Geometry: final body of the model. Coordinates: model frame, mm. A direction names the side the tool comes from. Give positions to 0.01 mm unless a question says otherwise; leave off trailing zeros. Loops run counter-clockwise (first coordinate to the right, second up) from the corner with the lowest first, then second, coordinate; pieces in that order, holes last.
from build123d import *

# Parameters (mm, degrees)
BOSS_EXTRUDE1_DEPTH = 20.5
SKETCH2_W           = 6
SKETCH2_H           = 13
SKETCH2_W_2         = 25
SKETCH2_H_2         = 6
CUT_EXTRUDE1_DEPTH  = 8
SKETCH3_W           = 23
SKETCH3_H           = 23
BOSS_EXTRUDE2_DEPTH = 7
SKETCH4_W           = 31
SKETCH4_H           = 32.5
SKETCH4_W_2         = 23
SKETCH4_H_2         = 23
BOSS_EXTRUDE4_DEPTH = 19
CUT_EXTRUDE2_REACH  = 53.403
SKETCH5_W           = 2.6
SKETCH5_H           = 5.5
SKETCH5_H_2         = 4
SKETCH5_W_2         = 4
SKETCH5_H_3         = 15
SKETCH5_W_3         = 2
SKETCH6_R           = 1.5
CUT_EXTRUDE3_DEPTH  = 10
SKETCH7_W           = 8
SKETCH7_H           = 9
BOSS_EXTRUDE5_DEPTH = 20.5
SKETCH8_R           = 2
CUT_EXTRUDE4_DEPTH  = 10


with BuildPart() as part:
    # Sketch1 → Boss-Extrude1 (new body)
    with BuildSketch(Plane(origin=(0, 0, 0), x_dir=(1, 0, 0), z_dir=(0, 1, 0))):
        Polygon((29, -32.5), (35, -32.5), (35, 32.5), (-35, 32.5), (-35, -32.5), (-29, -32.5), (-29, 26.5), (29, 26.5), align=None)
    extrude(amount=BOSS_EXTRUDE1_DEPTH)

    # Sketch2 → Cut-Extrude1 (cut)
    with BuildSketch(Plane.XZ):
        with Locations((32, 26)):
            Rectangle(SKETCH2_W, SKETCH2_H)
        with Locations((0, -29.5)):
            Rectangle(SKETCH2_W_2, SKETCH2_H_2)
        with Locations((-32, 26)):
            Rectangle(SKETCH2_W, SKETCH2_H)
    extrude(amount=-CUT_EXTRUDE1_DEPTH, mode=Mode.SUBTRACT)



with BuildPart() as body_2:
    # Sketch3 → Boss-Extrude2 (new body)
    with BuildSketch(Plane(origin=(0, 20.5, 0), x_dir=(1, 0, 0), z_dir=(0, 1, 0))):
        with Locations((-2.5, 9.5)):
            Rectangle(SKETCH3_W, SKETCH3_H)
    extrude(amount=-BOSS_EXTRUDE2_DEPTH)


with BuildPart() as part_1:
    add(part.part)

    add(body_2.part)  # Boss-Extrude4 merges body 2
    # Sketch4 → Boss-Extrude4 (add)
    with BuildSketch(Plane(origin=(0, 20.5, 0), x_dir=(1, 0, 0), z_dir=(0, 1, 0))):
        with Locations((-2.5, 10.25)):
            Rectangle(SKETCH4_W, SKETCH4_H)
        with Locations((-2.5, 9.5)):
            Rectangle(SKETCH4_W_2, SKETCH4_H_2, mode=Mode.SUBTRACT)
    extrude(amount=-BOSS_EXTRUDE4_DEPTH)

    # Cut-Extrude2: up to this face of the body (flat: up to its plane)
    cut_extrude2_end = Plane(part_1.part.faces().sort_by_distance((-2.5, 13.5, -9.5))[0])
    # Sketch5 → Cut-Extrude2 (cut, up to the picked face)
    with BuildSketch(Plane.XZ.offset(-1.5), mode=Mode.PRIVATE) as cut_extrude2_sk1:
        with Locations((-8.25, -23.75)):
            Rectangle(SKETCH5_W, SKETCH5_H)
    cut_extrude2_tool1 = split(extrude(cut_extrude2_sk1.sketch, amount=-CUT_EXTRUDE2_REACH, mode=Mode.PRIVATE), bisect_by=cut_extrude2_end, keep=Keep.BOTH, mode=Mode.PRIVATE)
    # Sketch5 → Cut-Extrude2 (cut, up to the picked face)
    with BuildSketch(Plane.XZ.offset(-1.5), mode=Mode.PRIVATE) as cut_extrude2_sk2:
        with Locations((-8.25, 4)):
            Rectangle(SKETCH5_W, SKETCH5_H_2)
    cut_extrude2_tool2 = split(extrude(cut_extrude2_sk2.sketch, amount=-CUT_EXTRUDE2_REACH, mode=Mode.PRIVATE), bisect_by=cut_extrude2_end, keep=Keep.BOTH, mode=Mode.PRIVATE)
    # Sketch5 → Cut-Extrude2 (cut, up to the picked face)
    with BuildSketch(Plane.XZ.offset(-1.5), mode=Mode.PRIVATE) as cut_extrude2_sk3:
        with Locations((-16, -5.5)):
            Rectangle(SKETCH5_W_2, SKETCH5_H_3)
    cut_extrude2_tool3 = split(extrude(cut_extrude2_sk3.sketch, amount=-CUT_EXTRUDE2_REACH, mode=Mode.PRIVATE), bisect_by=cut_extrude2_end, keep=Keep.BOTH, mode=Mode.PRIVATE)
    # Sketch5 → Cut-Extrude2 (cut, up to the picked face)
    with BuildSketch(Plane.XZ.offset(-1.5), mode=Mode.PRIVATE) as cut_extrude2_sk4:
        with Locations((3.55, 4)):
            Rectangle(SKETCH5_W_3, SKETCH5_H_2)
    cut_extrude2_tool4 = split(extrude(cut_extrude2_sk4.sketch, amount=-CUT_EXTRUDE2_REACH, mode=Mode.PRIVATE), bisect_by=cut_extrude2_end, keep=Keep.BOTH, mode=Mode.PRIVATE)
    add(cut_extrude2_tool1.solids().sort_by(Axis((-8.25, 1.5, -23.75), (0, 1, 0)))[0], mode=Mode.SUBTRACT)
    add(cut_extrude2_tool2.solids().sort_by(Axis((-8.25, 1.5, 4), (0, 1, 0)))[0], mode=Mode.SUBTRACT)
    add(cut_extrude2_tool3.solids().sort_by(Axis((-16, 1.5, -5.5), (0, 1, 0)))[0], mode=Mode.SUBTRACT)
    add(cut_extrude2_tool4.solids().sort_by(Axis((3.55, 1.5, 4), (0, 1, 0)))[0], mode=Mode.SUBTRACT)

    # Sketch6 → Cut-Extrude3 (cut)
    with BuildSketch(Plane.XZ):
        with Locations(Location((-32, 14.5, 0), (0, 0, 270))):
            Circle(SKETCH6_R)
        with Locations(Location((-32, -21.5, 0), (0, 0, 270))):
            Circle(SKETCH6_R)
    cut_extrude3 = extrude(amount=-CUT_EXTRUDE3_DEPTH, mode=Mode.SUBTRACT)

    # Mirror1: Cut-Extrude3 across plane
    add(cut_extrude3.mirror(Plane(origin=(0, 0, 0), x_dir=(0, 0, 1), z_dir=(1, 0, 0))), mode=Mode.SUBTRACT)

    # Sketch7 → Boss-Extrude5 (add)
    with BuildSketch(Plane(origin=(0, 20.5, 0), x_dir=(1, 0, 0), z_dir=(0, 1, 0))):
        with Locations((25, 22)):
            Rectangle(SKETCH7_W, SKETCH7_H)
        with Locations((-25, 22)):
            Rectangle(SKETCH7_W, SKETCH7_H)
    extrude(amount=-BOSS_EXTRUDE5_DEPTH)

    # Sketch8 → Cut-Extrude4 (cut)
    with BuildSketch(Plane(origin=(0, 0, -32.5), x_dir=(-1, 0, 0), z_dir=(0, 0, -1))):
        with Locations((-25, 11)):
            Circle(SKETCH8_R)
        with Locations((25, 11)):
            Circle(SKETCH8_R)
    extrude(amount=-CUT_EXTRUDE4_DEPTH, mode=Mode.SUBTRACT)


solid = part_1.part
Item 1: Section query A-A on z = 17.5. Return loops of the section in (x, y), plus the area to 3 significant figures.
Values follow:
outline: (-35, 0) - (-29, 0) - (-29, 20.5) - (-35, 20.5) - close; (29, 0) - (35, 0) - (35, 20.5) - (29, 20.5) - close
area: 246 mm2
Item 2: Section query D-D on x = 3.5. Return loops of the section in (y, z), plus the area to 4 significant figures.
Values follow:
outline: (1.5, -26.5) - (8, -26.5) - (8, -32.5) - (20.5, -32.5) - (20.5, 6) - (13.5, 6) - (13.5, -21) - (1.5, -21) - close
area: 368.5 mm2
Item 3: Pin query (flat end, axial travel): pin 1 (2 mm diameter, centred on x = -8, y = 11, fed in from +Z); pin 2 (6 mm diameter, centred on x = -22.5, y = 11, fed in from +Z); pin 3 (8 mm diameter, centred on x = -6.5, z = -5.5, fed in from -Y); pin 4 (10.5 mm diameter, centred on x = -3.5, y = 5, fed in from -Z). Return the tip coordinate at first contact, or that it passes through.
Values follow:
pin 1: stops at z = -26.5
pin 2: stops at z = -17.5
pin 3: stops at y = 13.5
pin 4: stops at z = -32.5
Item 4: Set-up query: faces 4 (the face through (-25, 11, -22.5)), 5 (the face through (-14, 7, 2)), 6 (the face through (3, 5, -26.5)), 7 (the face through (-29, 10, 8)). Return all of +Z, -Z, +X, -X, +Y, -Y with unobstructed straight access to the full face (end or side cutting, diameter ignored); none if empty.
Values follow:
face 4: -Z
face 5: -Y
face 6: -Z, -Y
face 7: +Z, +Y, -Y
Item 5: Draft query along Z for faces 1 (the face through (12.5, 4, -30)), 2 (the face through (-32, 10, -21)), 3 (the face through (-32, 14, 32.5)). Return one class per face: +Z half, -Z half, draft (parallel to the pull), parting line (faces both ways), or undercut.
Values follow:
face 1: draft
face 2: undercut
face 3: +Z half
Item 6: Section query B-B on y = 4.5. Give the number of separate pieces and of enclosed holes in the cut face, plus the area to 3 significant figures.
Values follow:
separate pieces: 4
enclosed holes: 4
area: 1,320 mm2
Item 7: Ray query, probe 1 along X at (y, z) = (3, 14.5); probe 2 along Z at (x, y) = (32, 5); probe 3 along Z at (x, y) = (-6.5, 9.25). Return the intervals inside material, ascending.
Values follow:
probe 1: x = -35 to -33.5, -30.5 to -29, 29 to 30.5, 33.5 to 35
probe 2: z = -32.5 to -23, -20 to 13, 16 to 19.5
probe 3: z = -32.5 to -21, 2 to 6
Item 8: Section query C-C on z = -3. Return loops of the section in (x, y).
Values follow:
outline: (-35, 0) - (-29, 0) - (-29, 20.5) - (-35, 20.5) - close; (-18, 13.5) - (9, 13.5) - (9, 1.5) - (13, 1.5) - (13, 20.5) - (-18, 20.5) - close; (29, 0) - (35, 0) - (35, 20.5) - (29, 20.5) - close
